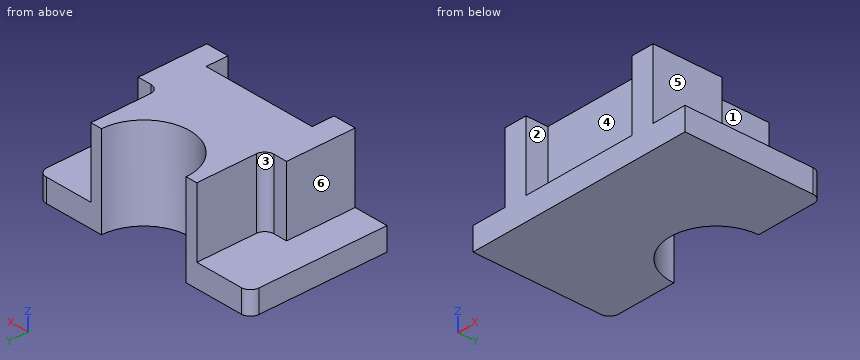
from build123d import *

# Parameters (mm, degrees)
F0_W      = 63.5
F0_H      = 38.1
F1_DEPTH  = 6.35
F2_W      = 44.45
F2_H      = 38.1
F3_DEPTH  = 19.05
F4_W      = 31.75
F4_H      = 12.158688
F5_DEPTH  = 19.05
F7_DEPTH  = 25.401
F9_W      = 6.35
F9_H      = 19.05
F10_DEPTH = 19.05
F11_W     = 6.35
F11_H     = 19.05
F12_DEPTH = 19.05
F13_R     = 2.54
F14_R     = 2.54
F15_R     = 2.54
F16_R     = 2.54


with BuildPart() as f1:
    # F0 (on Top) → F1 (new body)
    with BuildSketch(Plane.XY):
        Rectangle(F0_W, F0_H)
    extrude(amount=F1_DEPTH)

    # F2 (on face) → F3 (join)
    with BuildSketch(Plane.XY.offset(6.35)):
        Rectangle(F2_W, F2_H)
    extrude(amount=F3_DEPTH)

    # F4 (on face) → F5 (cut)
    with BuildSketch(Plane.XY.offset(25.4)):
        with Locations((0, -19.05)):
            Rectangle(F4_W, F4_H)
    extrude(amount=-F5_DEPTH, mode=Mode.SUBTRACT)

    # F6 (on face) → F7 (cut, through all)
    with BuildSketch(Plane.XY.offset(25.4)):
        with BuildLine():
            Line((-12.7, 19.05), (12.7, 19.05))
            ThreePointArc((12.7, 19.05), (0, 31.75), (-12.7, 19.05))
        make_face()
        with BuildLine():
            ThreePointArc((-12.7, 19.05), (0, 6.35), (12.7, 19.05))
            Line((12.7, 19.05), (-12.7, 19.05))
        make_face()
    extrude(amount=-F7_DEPTH, mode=Mode.SUBTRACT)

    # F9 (on face) → F10 (cut)
    with BuildSketch(Plane.XY.offset(25.4)):
        with Locations((-19.05, 9.525)):
            Rectangle(F9_W, F9_H)
    extrude(amount=-F10_DEPTH, mode=Mode.SUBTRACT)

    # F11 (on face) → F12 (cut)
    with BuildSketch(Plane.XY.offset(25.4)):
        with Locations((19.05, 9.525)):
            Rectangle(F11_W, F11_H)
    extrude(amount=-F12_DEPTH, mode=Mode.SUBTRACT)

    # F13
    f13_edges = [f1.edges().sort_by_distance(p)[0] for p in [
        (15.875, 0, 15.875),
    ]]
    fillet(f13_edges, radius=F13_R)

    # F14
    f14_edges = [f1.edges().sort_by_distance(p)[0] for p in [
        (-15.875, 0, 15.875),
    ]]
    fillet(f14_edges, radius=F14_R)

    # F15
    f15_edges = [f1.edges().sort_by_distance(p)[0] for p in [
        (-31.75, 19.05, 3.175),
    ]]
    fillet(f15_edges, radius=F15_R)

    # F16
    f16_edges = [f1.edges().sort_by_distance(p)[0] for p in [
        (31.75, 19.05, 3.175),
    ]]
    fillet(f16_edges, radius=F16_R)


solid = f1.part
Build history of the part. All positions in model axes, mm. Face numbers are marked on the shaded views. A direction names the side the tool comes from. Give positions to 0.01 mm unless a question says otherwise; leave off trailing zeros. Write each loop counter-clockwise with the first axis right and the second up, starting at its lowest first coordinate (ties: lowest second). Pieces come first, ordered by that corner, then holes. Notation, with made-up numbers: (-11, 0.5) - (9, 0.5) arc R35 cw to (9, 35.5) - close; hole circle Ø2 at (1, 22.25). An arc over 180 degrees is marked (long way). Use one line per item in the form item = value. Start each with the question number.
1. Band-saw the part on A-A on y = 4. Write the cut outline in (x, z) (3 decimals), plus the area to 3 significant figures.
2. 3-axis set-ups, long thin cutter, end or side, ignore diameter. For the marked faces 1, 2 and 3: which of +Z, -Z, +X, -X, +Y, -Y reach the whole face in a straight line?
3. Drop flat-ended pins along their axis: pin 1 Ø13 at (y, z) = (13.5, 14.5) entering from -X (3 decimals); pin 2 Ø1.1 at (x, z) = (-21, 20.5) entering from +Y; pin 3 Ø6.5 at (y, z) = (-14.5, 17.5) entering from +X (3 decimals). Give the stop position or say it passes through.
4. Probe line 1 (Y direction, x = -15, z = 21); line 2 (X direction, y = -1.5, z = 7.75) (3 decimals); line 3 (X direction, y = 2.5, z = 22.5). List the from-to ranges inside material, lowest first. Write a range as [from, to].
5. Band-saw the part on B-B on z = 2. Write the cut outline in (x, y).
6. Band-saw the part on C-C on x = 0. Write the cut outline in (y, z), plus the area to 3 significant figures.
7. Two-plate mould, pull along X, no slides. Class the marked faces 4, 5 and 6: released by +X, released by -X, zero draft, split by the parting line, or undercut.
8. Band-saw the part on D-D on y = 14. Write the cut outline in (x, z) (3 decimals), plus the area to 3 significant figures.
Conclusion:
q1.outline = (-31.75, 0) - (31.75, 0) - (31.75, 6.35) - (15.875, 6.35) - (15.875, 25.4) - (-15.875, 25.4) - (-15.875, 6.35) - (-31.75, 6.35) - close
q1.area = 1,010 mm²
q2.face_1 = +Z, +X, +Y
q2.face_2 = +Z, -Y
q2.face_3 = +Z, -X, +Y
q3.pin_1 = -15.875
q3.pin_2 = 0
q3.pin_3 = 22.225
q4.line_1 = [-12.97, 19.05]
q4.line_2 = [-22.225, 22.225]
q4.line_3 = [-15.88, 15.88]
q5.outline = (-31.75, -19.05) - (31.75, -19.05) - (31.75, 16.51) arc R2.54 ccw to (29.21, 19.05) - (12.7, 19.05) arc R12.7 cw to (-12.7, 19.05) - (-29.21, 19.05) arc R2.54 ccw to (-31.75, 16.51) - close
q6.outline = (-19.05, 0) - (6.35, 0) - (6.35, 25.4) - (-12.97, 25.4) - (-12.97, 6.35) - (-19.05, 6.35) - close
q6.area = 529 mm²
q7.face_4 = undercut
q7.face_5 = released by +X
q7.face_6 = released by -X
q8.outline = (-31.75, 0) - (-11.653, 0) - (-11.653, 25.4) - (-15.875, 25.4) - (-15.875, 6.35) - (-31.75, 6.35) - close; (11.653, 0) - (31.75, 0) - (31.75, 6.35) - (15.875, 6.35) - (15.875, 25.4) - (11.653, 25.4) - close
q8.area = 416 mm²
